Verification items for the finished model (mm, model axes). A direction names the side the tool comes from. Coordinates: 2 decimals unless noted, no trailing zeros. Write each loop counter-clockwise with the first axis right and the second up, starting at its lowest first coordinate (ties: lowest second). Pieces come first, ordered by that corner, then holes. Notation, with made-up numbers: M 23,21 L 66,21 A31 ccw 66,53 Z; hole C -23.75,28.25 d5. An arc over 180 degrees is marked long. Answer in a Markdown table with one row per item.
from build123d import *

# Parameters (mm, degrees)
F1_DEPTH = 10
F2_W     = 2.65
F2_H     = 2.65
F3_DEPTH = 2


with BuildPart() as f1:
    # F0 (on Front) → F1 (new body)
    with BuildSketch(Plane.XZ):
        Polygon((7.2, 0), (0, 0), (0, -50.5), (25.11394, 0), (16.01394, 0), (7.2, -18.62), align=None)
    extrude(amount=F1_DEPTH)

    # F2 (on face) → F3 (join)
    with BuildSketch(Plane.XY):
        with Locations((21.88894, -3.675)):
            Rectangle(F2_W, F2_H)
        with Locations((19.23894, -3.675)):
            Rectangle(F2_W, F2_H)
        with Locations((21.88894, -6.325)):
            Rectangle(F2_W, F2_H)
        with Locations((19.23894, -6.325)):
            Rectangle(F2_W, F2_H)
    extrude(amount=F3_DEPTH)


solid = f1.part
1) Release check for a two-part mould opening along X. For faces 5 (the face through (17.914, -5, 1)), 6 (the face through (7.2, -5, -9)), 7 (the face through (23.214, -5, 1)), 8 (the face through (4, -5, 0)) record: +X half, -X half, draft (parallel to the pull), parting line (faces both ways), or undercut.
Response values:
| item | result |
|---|---|
| face 5 | -X half |
| face 6 | undercut |
| face 7 | +X half |
| face 8 | draft |
2) Depth check by flat-ended pin: pin 1 (1.6 mm diameter, centred on x = 19.5, z = 1, fed in from -Y); pin 2 (1 mm diameter, centred on y = -4, z = 1.5, fed in from -X); pin 3 (0.6 mm diameter, centred on y = -4.5, z = 1, fed in from +X). Enter the tip coordinate at first touch or a pass-through.
Response values:
| item | result |
|---|---|
| pin 1 | stops at y = -7.65 |
| pin 2 | stops at x = 17.91 |
| pin 3 | stops at x = 23.21 |
3) Sectioned sample at A-A (z = -17.5). Record the cut outline in (x, y).
Response values:
| item | result |
|---|---|
| outline | M 0,-10 L 7.2,-10 L 7.2,0 L 0,0 Z; M 7.73,-10 L 16.41,-10 L 16.41,0 L 7.73,0 Z |
4) Sectioned sample at C-C (x = 20.5). Record the cut outline in (y, z), then the cut area to 3 significant figures.
Response values:
| item | result |
|---|---|
| outline | M -10,-9.28 L 0,-9.28 L 0,0 L -2.35,0 L -2.35,2 L -7.65,2 L -7.65,0 L -10,0 Z |
| area | 103 mm² |
5) Tool access check on faces 1 (the face through (11.67, -4.93, -9.18)), 2 (the face through (21, -2.35, 1)), 3 (the face through (21, -7.65, 1)), 4 (the face through (12.381, -4.93, -25.603)). Record the directions out of +Z, -Z, +X, -X, +Y, -Y that give a thin tool (end or side, any length) a straight path to the whole face; none if there is none.
Response values:
| item | result |
|---|---|
| face 1 | +Z, +Y, -Y |
| face 2 | +Z, +X, -X, +Y |
| face 3 | +Z, +X, -X, -Y |
| face 4 | -Z, +X, +Y, -Y |
6) Sectioned sample at B-B (y = -7). Record the cut outline in (x, z), then the cut area to 3 significant figures.
Response values:
| item | result |
|---|---|
| outline | M 0,-50.5 L 25.11,0 L 23.21,0 L 23.21,2 L 17.91,2 L 17.91,0 L 16.01,0 L 7.2,-18.62 L 7.2,0 L 0,0 Z |
| area | 563 mm² |
7) Sectioned sample at D-D (z = -7). Record the cut outline in (x, y).
Response values:
| item | result |
|---|---|
| outline | M 0,-10 L 7.2,-10 L 7.2,0 L 0,0 Z; M 12.7,-10 L 21.63,-10 L 21.63,0 L 12.7,0 Z |
8) Thickness scan on L1, parallel to X at y = -6.5, z = -7; L2, parallel to X at y = -7.25, z = -11.5; L3, parallel to Z at x = 13.5, y = -1.25. Record the ranges inside material, lowest first. Write a range as [from, to].
Response values:
| item | result |
|---|---|
| L1 | x = [0, 7.2], [12.7, 21.63] |
| L2 | x = [0, 7.2], [10.57, 19.39] |
| L3 | z = [-23.35, -5.31] |
